from build123d import *

# Parameters (mm, degrees)
SKETCH1_W           = 139.7
SKETCH1_H           = 203.2
BOSS_EXTRUDE1_DEPTH = 3.18
SKETCH2_R           = 1.5
SKETCH2_W           = 3.18
SKETCH2_H           = 91.725
CUT_EXTRUDE1_DEPTH  = 4.18
SKETCH3_R           = 8.441994665
CUT_EXTRUDE2_DEPTH  = 10
SKETCH5_W           = 25.530623926
SKETCH5_H           = 65.176444071
CUT_EXTRUDE3_DEPTH  = 10
SKETCH6_W           = 20.542742003
SKETCH6_H           = 14.404591712
BOSS_EXTRUDE2_DEPTH = 3.18
SKETCH7_W           = 56.63400571
SKETCH7_H           = 3.18
SKETCH7_W_2         = 56.95599429
CUT_EXTRUDE4_DEPTH  = 3.18
SKETCH8_W           = 3.18
SKETCH8_H           = 3.18
CUT_EXTRUDE5_DEPTH  = 80.56400571


with BuildPart() as part:
    # Sketch1 → Boss-Extrude1 (new body)
    with BuildSketch(Plane.XY):
        Rectangle(SKETCH1_W, SKETCH1_H)
    extrude(amount=BOSS_EXTRUDE1_DEPTH)

    # Sketch2 → Cut-Extrude1 (cut, through all)
    with BuildSketch(Plane.XY.offset(3.18)):
        with Locations((-67.85, 0)):
            Circle(SKETCH2_R)
        with Locations((67.85, 0)):
            Circle(SKETCH2_R)
        Polygon((-10, 101.6), (10, 101.6), (10, 98.42), (1.5, 98.42), (1.5, 94.42), (3.5, 94.42), (3.5, 91.42), (1.5, 91.42), (1.5, 88.42), (-1.5, 88.42), (-1.5, 91.42), (-3.5, 91.42), (-3.5, 94.42), (-1.5, 94.42), (-1.5, 98.42), (-10, 98.42), align=None)
        Polygon((-10, -101.6), (-10, -98.42), (-1.5, -98.42), (-1.5, -94.42), (-3.5, -94.42), (-3.5, -91.42), (-1.5, -91.42), (-1.5, -88.42), (1.5, -88.42), (1.5, -91.42), (3.5, -91.42), (3.5, -94.42), (1.5, -94.42), (1.5, -98.42), (10, -98.42), (10, -101.6), align=None)
        with Locations((-68.26, 55.7375)):
            Rectangle(SKETCH2_W, SKETCH2_H)
        with Locations((-68.26, -55.7375)):
            Rectangle(SKETCH2_W, SKETCH2_H)
        with Locations((68.26, -55.7375)):
            Rectangle(SKETCH2_W, SKETCH2_H)
        with Locations((68.26, 55.7375)):
            Rectangle(SKETCH2_W, SKETCH2_H)
    extrude(amount=-CUT_EXTRUDE1_DEPTH, mode=Mode.SUBTRACT)

    # Sketch3 → Cut-Extrude2 (cut)
    with BuildSketch(Plane(origin=(0, 0, 0), x_dir=(-1, 0, 0), z_dir=(0, 0, -1))):
        with Locations((0.068813102, -81.648638462)):
            Circle(SKETCH3_R)
    extrude(amount=-CUT_EXTRUDE2_DEPTH, mode=Mode.SUBTRACT)

    # Sketch5 → Cut-Extrude3 (cut)
    with BuildSketch(Plane(origin=(0, 0, 0), x_dir=(-1, 0, 0), z_dir=(0, 0, -1))):
        with Locations((0, 52.074409839)):
            Rectangle(SKETCH5_W, SKETCH5_H)
    extrude(amount=-CUT_EXTRUDE3_DEPTH, mode=Mode.SUBTRACT)

    # Sketch6 → Boss-Extrude2 (add)
    with BuildSketch(Plane(origin=(0, 0, 0), x_dir=(-1, 0, 0), z_dir=(0, 0, -1))):
        with Locations((0.271371002, 94.397704144)):
            Rectangle(SKETCH6_W, SKETCH6_H)
    extrude(amount=-BOSS_EXTRUDE2_DEPTH)

    # Sketch7 → Cut-Extrude4 (cut)
    with BuildSketch(Plane(origin=(0, 0, 0), x_dir=(-1, 0, 0), z_dir=(0, 0, -1))):
        with Locations((-38.352997145, 100.01)):
            Rectangle(SKETCH7_W, SKETCH7_H)
        with Locations((38.192002855, 100.01)):
            Rectangle(SKETCH7_W_2, SKETCH7_H)
    extrude(amount=-CUT_EXTRUDE4_DEPTH, mode=Mode.SUBTRACT)

    # Sketch8 → Cut-Extrude5 (cut, through all)
    with BuildSketch(Plane.ZY.offset(9.71400571)):
        with Locations((1.59, 100.01)):
            Rectangle(SKETCH8_W, SKETCH8_H)
    extrude(amount=-CUT_EXTRUDE5_DEPTH, mode=Mode.SUBTRACT)


solid = part.part
Work out the finished part from the listing and answer in its coordinate system (mm). Give positions to 0.01 mm unless a question says otherwise; leave off trailing zeros. Loops run counter-clockwise (first coordinate to the right, second up) from the corner with the lowest first, then second, coordinate; pieces in that order, holes last. Notation, with made-up numbers: (6, 16) -> (64, 16) arc R27 ccw to (64, 49) -> close; hole circle Ø2 at (41.25, -9). An arc over 180 degrees is marked (long way). Use a Markdown table: item, result. Add a question column.
1) The part is cut by section B-B, the plane y = 15. Determine the outline of the cut face in (x, z), plus the area to 3 significant figures.
2) For a pull along X with two mould halves and no side action, classify faces 1 (the flat face through (-1, 0, 3.18)), 2 (the cylindrical face through (-0.489, -73.217, 1.568)) as +X half, -X half, draft (parallel to the pull), parting line (faces both ways), or undercut.
3) The part is cut by section A-A, the plane z = 1. Count the separate pieces of the cut face and the enclosed holes in it, plus the area to 3 significant figures.
4) Consider line 1 along X through (y, z) = (41, 0.3); line 2 along Y through (x, z) = (-67.85, 0.6) (3 decimals); line 3 along X through (y, z) = (-13, 1.25). Determine where each line is inside the solid, lowest interval first.
5) Each of these flat-tipped pins is pushed along its axis until it touches: P1, Ø1, axis at y = -100.5, z = 1, coming from the -X side; P2, Ø15, axis at x = -0.07, y = -81.65, coming from the +Z side; P3, Ø1, axis at y = 69.5, z = 2, coming from the +X side; P4, Ø1.6, axis at x = 4, z = 1.5, coming from the -Y side. Where does it stop, or does it pass through?
Reported:
| question | item | result |
|---|---|---|
| 1 | outline | (-66.67, 0) -> (66.67, 0) -> (66.67, 3.18) -> (-66.67, 3.18) -> close |
| 1 | area | 424 mm^2 |
| 2 | face 1 | draft |
| 2 | face 2 | undercut |
| 3 | separate pieces | 1 |
| 3 | enclosed holes | 3 |
| 3 | area | 24,800 mm^2 |
| 4 | line 1 | x = -66.67 to -12.77, 12.77 to 66.67 |
| 4 | line 2 | y = -9.875 to -1.5, 1.5 to 9.875 |
| 4 | line 3 | x = -66.67 to 66.67 |
| 5 | P1 | stops at x = -66.67 |
| 5 | P2 | passes through |
| 5 | P3 | stops at x = 66.67 |
| 5 | P4 | stops at y = -98.42 |
